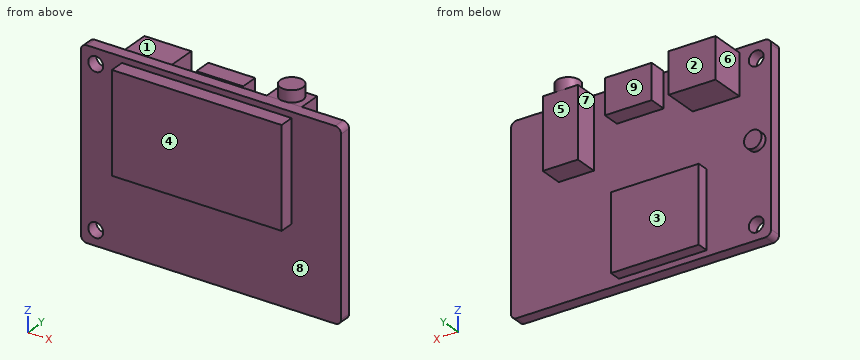
from build123d import *

# Parameters (mm, degrees)
SKETCH1_W           = 44.45
SKETCH1_H           = 31.75
BOSS_EXTRUDE1_DEPTH = 2
SKETCH2_R           = 1.27
CUT_EXTRUDE1_DEPTH  = 2
FILLET1_R           = 1
FILLET2_R           = 1
FILLET3_R           = 1
FILLET4_R           = 1
SKETCH3_W           = 8
SKETCH3_H           = 7
BOSS_EXTRUDE2_DEPTH = 6
SKETCH4_W           = 8
SKETCH4_H           = 6
BOSS_EXTRUDE3_DEPTH = 3
SKETCH5_W           = 6
SKETCH5_H           = 12
BOSS_EXTRUDE4_DEPTH = 4
SKETCH6_R           = 1.95
BOSS_EXTRUDE5_DEPTH = 2
SKETCH7_R           = 1.5
BOSS_EXTRUDE6_DEPTH = 1
SKETCH9_W           = 15
SKETCH9_H           = 13
BOSS_EXTRUDE7_DEPTH = 2
SKETCH10_W          = 29
SKETCH10_H          = 17
BOSS_EXTRUDE8_DEPTH = 2.5


with BuildPart() as part:
    # Sketch1 → Boss-Extrude1 (new body)
    with BuildSketch(Plane(origin=(0, 0, 0), x_dir=(1, 0, 0), z_dir=(0, 1, 0))):
        Rectangle(SKETCH1_W, SKETCH1_H)
    extrude(amount=BOSS_EXTRUDE1_DEPTH)

    # Sketch2 → Cut-Extrude1 (cut)
    with BuildSketch(Plane(origin=(0, 2, 0), x_dir=(1, 0, 0), z_dir=(0, 1, 0))):
        with Locations((-19.685, -13.335)):
            Circle(SKETCH2_R)
        with Locations((-19.685, 13.335)):
            Circle(SKETCH2_R)
    extrude(amount=-CUT_EXTRUDE1_DEPTH, mode=Mode.SUBTRACT)

    # Fillet1
    fillet1_edges = [part.edges().sort_by_distance(p)[0] for p in [
        (-22.225, 1, -15.875),
    ]]
    fillet(fillet1_edges, radius=FILLET1_R)

    # Fillet2
    fillet2_edges = [part.edges().sort_by_distance(p)[0] for p in [
        (-22.225, 1, 15.875),
    ]]
    fillet(fillet2_edges, radius=FILLET2_R)

    # Fillet3
    fillet3_edges = [part.edges().sort_by_distance(p)[0] for p in [
        (22.225, 1, -15.875),
    ]]
    fillet(fillet3_edges, radius=FILLET3_R)

    # Fillet4
    fillet4_edges = [part.edges().sort_by_distance(p)[0] for p in [
        (22.225, 1, 15.875),
    ]]
    fillet(fillet4_edges, radius=FILLET4_R)

    # Sketch3 → Boss-Extrude2 (add)
    with BuildSketch(Plane(origin=(0, 2, 0), x_dir=(1, 0, 0), z_dir=(0, 1, 0))):
        with Locations((-12.827, -11.625)):
            Rectangle(SKETCH3_W, SKETCH3_H)
    extrude(amount=BOSS_EXTRUDE2_DEPTH)

    # Sketch4 → Boss-Extrude3 (add)
    with BuildSketch(Plane(origin=(0, 2, 0), x_dir=(1, 0, 0), z_dir=(0, 1, 0))):
        with Locations((0.127, -13.125)):
            Rectangle(SKETCH4_W, SKETCH4_H)
    extrude(amount=BOSS_EXTRUDE3_DEPTH)

    # Sketch5 → Boss-Extrude4 (add)
    with BuildSketch(Plane(origin=(0, 2, 0), x_dir=(1, 0, 0), z_dir=(0, 1, 0))):
        with Locations((11.049, -9.775)):
            Rectangle(SKETCH5_W, SKETCH5_H)
    extrude(amount=BOSS_EXTRUDE4_DEPTH)

    # Sketch6 → Boss-Extrude5 (add)
    with BuildSketch(Plane.XY.offset(15.775)):
        with Locations((11.049, 4)):
            Circle(SKETCH6_R)
    extrude(amount=BOSS_EXTRUDE5_DEPTH)

    # Sketch7 → Boss-Extrude6 (add)
    with BuildSketch(Plane(origin=(0, 2, 0), x_dir=(1, 0, 0), z_dir=(0, 1, 0))):
        with Locations((-19.775, 0.125)):
            Circle(SKETCH7_R)
    extrude(amount=BOSS_EXTRUDE6_DEPTH)

    # Sketch9 → Boss-Extrude7 (add)
    with BuildSketch(Plane(origin=(0, 2, 0), x_dir=(1, 0, 0), z_dir=(0, 1, 0))):
        with Locations((-3.725, 8.375)):
            Rectangle(SKETCH9_W, SKETCH9_H)
    extrude(amount=BOSS_EXTRUDE7_DEPTH)

    # Sketch10 → Boss-Extrude8 (add)
    with BuildSketch(Plane.XZ):
        with Locations((-0.725, 6.375)):
            Rectangle(SKETCH10_W, SKETCH10_H)
    extrude(amount=BOSS_EXTRUDE8_DEPTH)


solid = part.part
Check sheet for the modelled part. Datum: model origin and axes. Units: mm. Face numbers are marked on the shaded views. A direction names the side the tool comes from. Give positions to 0.01 mm unless a question says otherwise; leave off trailing zeros. Write each loop counter-clockwise with the first axis right and the second up, starting at its lowest first coordinate (ties: lowest second). Pieces come first, ordered by that corner, then holes. Notation, with made-up numbers: (20, 41.5) -> (72, 41.5) arc R26 cw to (72, 70.5) -> close; hole circle Ø8 at (76.5, -21.75). An arc over 180 degrees is marked (long way). One line per item, written item: value. Start each with the question number.
Item 1: Section check A-A on z = 11.5. Record the cut outline in (x, y) (3 decimals).
Item 2: Tool access check on the marked faces 1, 2, 3, 4 and 5. Record the directions out of +Z, -Z, +X, -X, +Y, -Y that give a thin tool (end or side, any length) a straight path to the whole face; none if there is none.
Item 3: Draft check along X on the marked faces 6, 7, 8 and 9. Enter one of: +X half, -X half, draft (parallel to the pull), parting line (faces both ways), or undercut.
Item 4: Section check B-B on x = 17. Record the cut outline in (y, z) (3 decimals), then the cut area to 3 significant figures.
Item 5: Gauge pin test, flat ends, axial feed: pin 1 (1.6 mm diameter, centred on y = 3.5, z = -9, fed in from +X) (3 decimals); pin 2 (1.6 mm diameter, centred on x = -4.5, y = 3, fed in from +Z) (3 decimals); pin 3 (1.5 mm diameter, centred on x = -4, z = -11, fed in from +Y). Record the tip position at first contact, or that the pin passes through.
Item 6: Material ranges on probe 1 along X at (y, z) = (3.75, 12); probe 2 along Y at (x, z) = (12, 13); probe 3 along Y at (x, z) = (-3, 10.5), recorded low to high. Write a range as from..to.
Results list:
1. outline: (-22.225, 0) -> (-15.225, 0) -> (-15.225, -2.5) -> (13.775, -2.5) -> (13.775, 0) -> (22.225, 0) -> (22.225, 2) -> (14.049, 2) -> (14.049, 6) -> (8.049, 6) -> (8.049, 2) -> (4.127, 2) -> (4.127, 5) -> (-3.873, 5) -> (-3.873, 2) -> (-8.827, 2) -> (-8.827, 8) -> (-16.827, 8) -> (-16.827, 2) -> (-22.225, 2) -> close
2. face 1: +Z, -X, +Y
2. face 2: +Z, -Z, +X, -X, +Y
2. face 3: -Z, +X, -X, +Y
2. face 4: +Z, -Z, +X, -X, -Y
2. face 5: +Z, -Z, +X, +Y
3. face 6: -X half
3. face 7: undercut
3. face 8: draft
3. face 9: undercut
4. outline: (0, -15.875) -> (2, -15.875) -> (2, 15.875) -> (0, 15.875) -> close
4. area: 63.5 mm²
5. pin 1: x = 3.775
5. pin 2: z = 16.125
5. pin 3: y = 4
6. probe 1: -16.83..-8.83, -3.87..4.13, 8.05..14.05
6. probe 2: -2.5..6
6. probe 3: -2.5..5
